Model file for the job. Use its own axes, mm. A direction names the side the tool comes from. Coordinates: 2 decimals unless noted, no trailing zeros. Loops run counter-clockwise (first coordinate to the right, second up) from the corner with the lowest first, then second, coordinate; pieces in that order, holes last. Notation, with made-up numbers: (31.25, -16) -> (79.25, -16) arc R20 cw to (79.25, 20) -> close; hole circle Ø4 at (-7.5, -21). An arc over 180 degrees is marked (long way). Use one line per item in the form item = value.
```python
from build123d import *

# Parameters (mm, degrees)
SKETCH1_W           = 17
SKETCH1_H           = 32
SKETCH1_R           = 2.5
BOSS_EXTRUDE1_DEPTH = 5
SKETCH2_R           = 6
SKETCH2_R_2         = 4.025
BOSS_EXTRUDE2_DEPTH = 15
FILLET1_R           = 1


with BuildPart() as part:
    # Sketch1 → Boss-Extrude1 (new body)
    with BuildSketch(Plane(origin=(0, 0, 0), x_dir=(1, 0, 0), z_dir=(0, 1, 0))):
        Rectangle(SKETCH1_W, SKETCH1_H)
        with Locations(Location((0, 11.5, 0), (0, 0, 270))):
            Circle(SKETCH1_R, mode=Mode.SUBTRACT)
        with Locations(Location((0, -11.5, 0), (0, 0, 270))):
            Circle(SKETCH1_R, mode=Mode.SUBTRACT)
    extrude(amount=BOSS_EXTRUDE1_DEPTH)

    # Sketch2 → Boss-Extrude2 (add)
    with BuildSketch(Plane(origin=(0, 5, 0), x_dir=(1, 0, 0), z_dir=(0, 1, 0))):
        with Locations(Location((0, 0, 0), (0, 0, 90))):
            Circle(SKETCH2_R)
        with Locations(Location((0, 0, 0), (0, 0, 270))):
            Circle(SKETCH2_R_2, mode=Mode.SUBTRACT)
    extrude(amount=BOSS_EXTRUDE2_DEPTH)

    # Fillet1
    fillet1_edges = [part.edges().sort_by_distance(p)[0] for p in [
        (-8.5, 5, 0),
        (0, 5, 16),
        (8.5, 5, 0),
        (0, 5, -16),
    ]]
    fillet(fillet1_edges, radius=FILLET1_R)


solid = part.part
```
Q1. Band-saw the part on C-C, the plane z = 0. Write the cut outline in (x, y) (3 decimals), and give its area (3 significant figures).
Result:
outline = (-8.5, 0) -> (8.5, 0) -> (8.5, 4) arc R1 ccw to (7.5, 5) -> (6, 5) -> (6, 20) -> (4.025, 20) -> (4.025, 5) -> (-4.025, 5) -> (-4.025, 20) -> (-6, 20) -> (-6, 5) -> (-7.5, 5) arc R1 ccw to (-8.5, 4) -> close
area = 144 mm2
Q2. Wall check: line 1 along X through (y, z) = (3.25, -11.5); line 2 along X through (y, z) = (14.75, 0) (3 decimals); line 3 along Y through (x, z) = (-4, -12). Give the ranges that are in metal, low to high.
Result:
line_1 = -8.5 to -2.5, 2.5 to 8.5
line_2 = -6 to -4.025, 4.025 to 6
line_3 = 0 to 5
Q3. Which spindle directions (+Z, -Z, +X, -X, +Y, -Y) get a long thin tool onto all of the face, cutting with end or side? Do faces 5 (the face through (0.119, 4.699, -15.715)), 6 (the face through (-1.802, 12.395, -5.723)). Say none if no direction does.
Result:
face_5 = -Z, +X, -X, +Y
face_6 = +Y
Q4. Band-saw the part on B-B, the plane z = -11.5. Write the cut outline in (x, y).
Result:
outline = (-8.5, 0) -> (-2.5, 0) -> (-2.5, 5) -> (-7.5, 5) arc R1 ccw to (-8.5, 4) -> close; (2.5, 0) -> (8.5, 0) -> (8.5, 4) arc R1 ccw to (7.5, 5) -> (2.5, 5) -> close
Q5. Band-saw the part on D-D, the plane x = -7. Write the cut outline in (y, z), and give its area (3 significant figures).
Result:
outline = (0, -16) -> (4, -16) arc R1 ccw to (5, -15) -> (5, 15) arc R1 ccw to (4, 16) -> (0, 16) -> close
area = 160 mm2
Q6. Pin check, flat tips, straight feed: pin 1 Ø4 at (x, y) = (-3.5, 8.5) entering from +Z; pin 2 Ø5 at (y, z) = (15, 6) entering from -X; pin 3 Ø4 at (x, y) = (2.5, 8.5) entering from -Z; pin 4 Ø9.5 at (x, z) = (0, 0) entering from +Y. Stop position of each tip, or through.
Result:
pin_1 = 5.81
pin_2 = -4.87
pin_3 = -5.98
pin_4 = 20
Q7. Band-saw the part on A-A, the plane x = 0. Write the cut outline in (y, z) (3 decimals).
Result:
outline = (0, -16) -> (4, -16) arc R1 ccw to (5, -15) -> (5, -14) -> (0, -14) -> close; (0, -9) -> (5, -9) -> (5, -6) -> (20, -6) -> (20, -4.025) -> (5, -4.025) -> (5, 4.025) -> (20, 4.025) -> (20, 6) -> (5, 6) -> (5, 9) -> (0, 9) -> close; (0, 14) -> (5, 14) -> (5, 15) arc R1 ccw to (4, 16) -> (0, 16) -> close
Q8. Mould opens along X. For faces 1 (the face through (8.199, 4.715, -0.224)), 2 (the face through (0, 5, 0)), 3 (the face through (-8.5, 2, 0)), 4 (the face through (0, 2, 16)) say: released by +X, released by -X, zero draft, split by the parting line, or undercut.
Result:
face_1 = released by +X
face_2 = undercut
face_3 = released by -X
face_4 = zero draft
